Part model, mm, in its own coordinate system. Face numbers are marked on the shaded views. Coordinates: 2 decimals unless noted, no trailing zeros. Write each loop counter-clockwise with the first axis right and the second up, starting at its lowest first coordinate (ties: lowest second). Pieces come first, ordered by that corner, then holes. Notation, with made-up numbers: (22, 11.25) - (59, 11.25) arc R32 cw to (59, 41.25) - close; hole circle Ø6 at (49.5, -8.75). An arc over 180 degrees is marked (long way). Use a Markdown table: item, result.
```python
from build123d import *

# Parameters (mm, degrees)
F0_R     = 3.0353
F0_R_2   = 19.177
F0_R_3   = 30
F1_DEPTH = 25.4


with BuildPart() as f1:
    # F0 (on Top) → F1 (new body)
    with BuildSketch(Plane.XY):
        with BuildLine():
            ThreePointArc((-31.291722, -68.875), (0, -95.25), (31.291722, -68.875))
            Line((31.291722, -68.875), (41.886557, -7.194882))
            ThreePointArc((41.886557, -7.194882), (0, 42.5), (-41.886557, -7.194882))
            Line((-41.886557, -7.194882), (-31.291722, -68.875))
        make_face()
        with Locations((0, -88.9)):
            Circle(F0_R, mode=Mode.SUBTRACT)
        with Locations((0, -63.5)):
            Circle(F0_R_2, mode=Mode.SUBTRACT)
        with Locations((0, -36.2458)):
            Circle(F0_R, mode=Mode.SUBTRACT)
        with Locations((-36.2458, 0)):
            Circle(F0_R, mode=Mode.SUBTRACT)
        Circle(F0_R_3, mode=Mode.SUBTRACT)
        with Locations((36.2458, 0)):
            Circle(F0_R, mode=Mode.SUBTRACT)
        with Locations((0, 36.2458)):
            Circle(F0_R, mode=Mode.SUBTRACT)
    extrude(amount=F1_DEPTH)


solid = f1.part
```
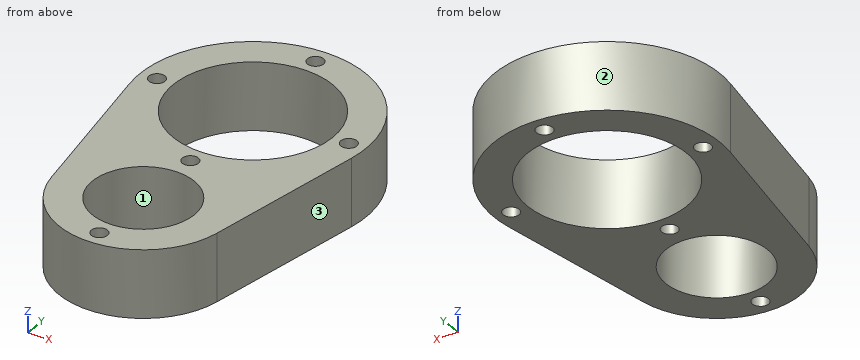
Item 1: Band-saw the part on B-B, the plane y = 0. Give the cut face in (x, z), then the cut area to 3 significant figures.
From the geometry:
| item | result |
|---|---|
| outline | (-42.5, 0) - (-39.28, 0) - (-39.28, 25.4) - (-42.5, 25.4) - close; (-33.21, 0) - (-30, 0) - (-30, 25.4) - (-33.21, 25.4) - close; (30, 0) - (33.21, 0) - (33.21, 25.4) - (30, 25.4) - close; (39.28, 0) - (42.5, 0) - (42.5, 25.4) - (39.28, 25.4) - close |
| area | 327 mm^2 |
Item 2: Band-saw the part on C-C, the plane y = -88.9. Give the cut face in (x, z), then the cut area to 3 significant figures.
From the geometry:
| item | result |
|---|---|
| outline | (-19.05, 0) - (-3.04, 0) - (-3.04, 25.4) - (-19.05, 25.4) - close; (3.04, 0) - (19.05, 0) - (19.05, 25.4) - (3.04, 25.4) - close |
| area | 814 mm^2 |
Item 3: Band-saw the part on A-A, the plane x = 0. Give the cut face in (y, z).
From the geometry:
| item | result |
|---|---|
| outline | (-95.25, 0) - (-91.94, 0) - (-91.94, 25.4) - (-95.25, 25.4) - close; (-85.86, 0) - (-82.68, 0) - (-82.68, 25.4) - (-85.86, 25.4) - close; (-44.32, 0) - (-39.28, 0) - (-39.28, 25.4) - (-44.32, 25.4) - close; (-33.21, 0) - (-30, 0) - (-30, 25.4) - (-33.21, 25.4) - close; (30, 0) - (33.21, 0) - (33.21, 25.4) - (30, 25.4) - close; (39.28, 0) - (42.5, 0) - (42.5, 25.4) - (39.28, 25.4) - close |
Item 4: Two-plate mould, pull along X, no slides. Class the marked faces 1, 2 and 3: pulls with the +X half, pulls with the -X half, needs draft (parallel to the pull), parting line crosses it, or undercut.
From the geometry:
| item | result |
|---|---|
| face 1 | undercut |
| face 2 | parting line crosses it |
| face 3 | pulls with the +X half |
Item 5: Drop flat-ended pins along their axis: P1, Ø5, axis at x = 28.5, z = 22, coming from the -Y side; P2, Ø8, axis at y = 23.5, z = 7, coming from the -X side; P3, Ø12, axis at y = -21.5, z = 9.5, coming from the -X side. Give the stop position or say it passes through.
From the geometry:
| item | result |
|---|---|
| P1 | y = -81.72 |
| P2 | x = -37.76 |
| P3 | x = -40.46 |
Item 6: Drill centre lines: probe 1 along Y at (x, z) = (17, 21); probe 2 along Y at (x, z) = (10.5, 10.5); probe 3 along X at (y, z) = (-79, 10.25). Where is each one in solid material? Low to high.
From the geometry:
| item | result |
|---|---|
| probe 1 | -90.32 to -72.37, -54.63 to -24.72, 24.72 to 38.95 |
| probe 2 | -93.46 to -79.55, -47.45 to -28.1, 28.1 to 41.18 |
| probe 3 | -27.71 to -11.29, 11.29 to 27.71 |
Item 7: Band-saw the part on D-D, the plane z = 6. Count the separate pieces of the cut face and the enclosed holes in it, then the cut area to 3 significant figures.
From the geometry:
| item | result |
|---|---|
| separate pieces | 1 |
| enclosed holes | 7 |
| area | 5,080 mm^2 |
